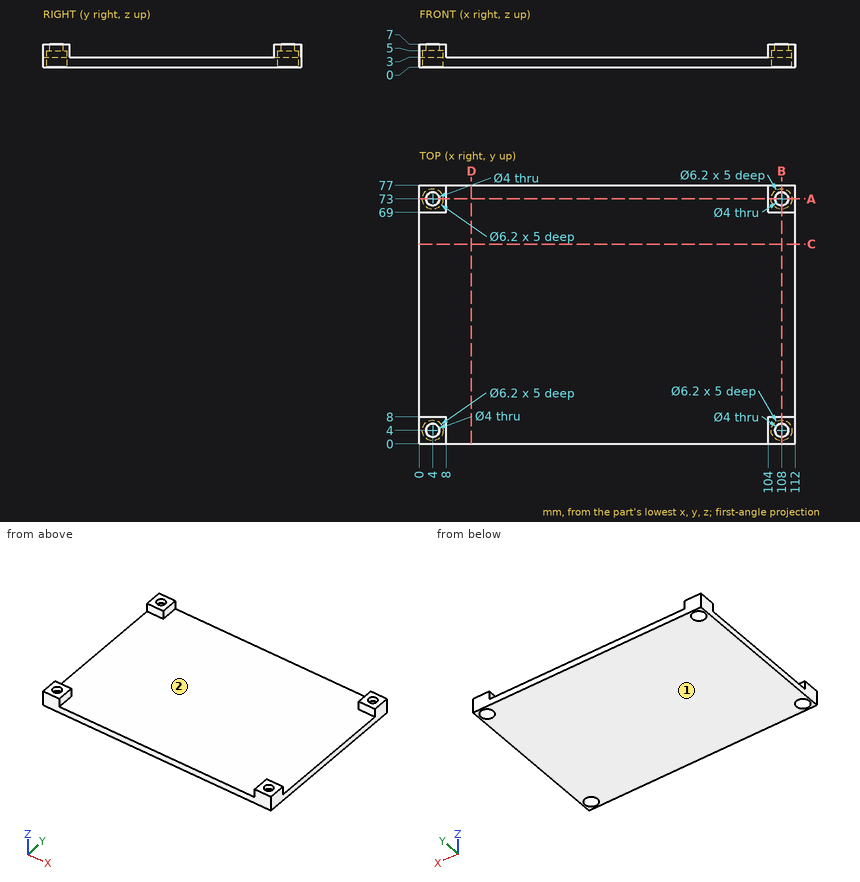
Here's the drawing with two shaded views (mm, measured from the low corner). I have some questions. Give positions to 0.01 mm unless a question says otherwise; leave off trailing zeros. Order: outer loops, then holes, each group sorted by start corner. A loop starts at its lowest first (then second) coordinate and runs counter-clockwise, first axis right, second up. Notation, with made-up numbers: (-37, 87.5) -> (17, 87.5) arc R23 cw to (17, 106.5) -> close; hole circle Ø5 at (0, -23). An arc over 180 degrees is marked (long way). Use a Markdown table: item, result. Add a question column.
Item 1: I need wall thicknesses on line 1 (Y direction, x = 108, z = 2.65); line 2 (Y direction, x = 108, z = 6.55); line 3 (X direction, y = 4, z = 1.55). Which ranges of each line are inside material? Lowest first, please.
Item 2: Imagine slicing it at A-A on y = 73. Please give me the cut outline in (x, z).
Item 3: Imagine slicing it at D-D on x = 15.5. Please give me the cut outline in (y, z).
Item 4: Will these pins go through, and if not, where does the flat tip stop? pin 1 (7 mm diameter, centred on x = 108.5, y = 73, fed in from -Z); pin 2 (1.9 mm diameter, centred on x = 3, y = 74, fed in from -Z); pin 3 (23 mm diameter, centred on x = 76.5, y = 38, fed in from +Z).
Item 5: If we mould it in two halves opening along X, with no side actions, what happens to the marked faces 1 and 2? For each: pulls with the +X half, pulls with the -X half, needs draft (parallel to the pull), parting line crosses it, or undercut.
Item 6: Imagine slicing it at C-C on y = 59.5. Please give me the cut outline in (x, z).
Item 7: Imagine slicing it at B-B on x = 108. Please give me the cut outline in (y, z), plus the area to 3 significant figures.
Data:
| question | item | result |
|---|---|---|
| 1 | line 1 | y = 0 to 0.9, 7.1 to 69.9, 76.1 to 77 |
| 1 | line 2 | y = 0 to 2, 6 to 8, 69 to 71, 75 to 77 |
| 1 | line 3 | x = 0 to 0.9, 7.1 to 104.9, 111.1 to 112 |
| 2 | outline | (0, 0) -> (0.9, 0) -> (0.9, 5) -> (2, 5) -> (2, 7) -> (0, 7) -> close; (6, 5) -> (7.1, 5) -> (7.1, 0) -> (104.9, 0) -> (104.9, 5) -> (106, 5) -> (106, 7) -> (104, 7) -> (104, 3) -> (8, 3) -> (8, 7) -> (6, 7) -> close; (110, 5) -> (111.1, 5) -> (111.1, 0) -> (112, 0) -> (112, 7) -> (110, 7) -> close |
| 3 | outline | (0, 0) -> (77, 0) -> (77, 3) -> (0, 3) -> close |
| 4 | pin 1 | stops at z = 0 |
| 4 | pin 2 | stops at z = 5 |
| 4 | pin 3 | stops at z = 3 |
| 5 | face 1 | needs draft |
| 5 | face 2 | undercut |
| 6 | outline | (0, 0) -> (112, 0) -> (112, 3) -> (0, 3) -> close |
| 7 | outline | (0, 0) -> (0.9, 0) -> (0.9, 5) -> (2, 5) -> (2, 7) -> (0, 7) -> close; (6, 5) -> (7.1, 5) -> (7.1, 0) -> (69.9, 0) -> (69.9, 5) -> (71, 5) -> (71, 7) -> (69, 7) -> (69, 3) -> (8, 3) -> (8, 7) -> (6, 7) -> close; (75, 5) -> (76.1, 5) -> (76.1, 0) -> (77, 0) -> (77, 7) -> (75, 7) -> close |
| 7 | area | 217 mm² |
